Source: CAD feature listing. Evaluate the final solid. Frame: model axes, mm. A direction names the side the tool comes from. Coordinates: 2 decimals unless noted, no trailing zeros. Order: outer loops, then holes, each group sorted by start corner. A loop starts at its lowest first (then second) coordinate and runs counter-clockwise, first axis right, second up.
```python
from build123d import *

# Parameters (mm, degrees)
F0_R     = 25.4
F1_DEPTH = 635
F2_W     = 63.5
F2_H     = 50.8
F3_DEPTH = 25.4
F4_R     = 5.08


with BuildPart() as f1:
    # F0 (on Top) → F1 (new body)
    with BuildSketch(Plane.XY):
        Circle(F0_R)
    extrude(amount=F1_DEPTH)

    # F2 (on Front) → F3 (cut)
    with BuildSketch(Plane.XZ):
        with Locations((0.1835199598, 25.4)):
            Rectangle(F2_W, F2_H)
    extrude(amount=-F3_DEPTH, mode=Mode.SUBTRACT)

    # F4
    f4_edges = [f1.edges().sort_by_distance(p)[0] for p in [
        (-25.4, 0, 635),
    ]]
    fillet(f4_edges, radius=F4_R)


solid = f1.part
```
1. Pin query (flat end, axial travel): P1, Ø12, axis at y = -7.5, z = 66.5, coming from the +X side; P2, Ø4, axis at x = -20, z = 79, coming from the -Y side; P3, Ø2, axis at y = -3.5, z = 315.5, coming from the +X side. Return the tip coordinate at first contact, or that it passes through.
Findings:
P1: stops at x = 25.36
P2: stops at y = -17.92
P3: stops at x = 25.28
2. Ray query, line 1 (X direction, y = -2.5, z = 368.5); line 2 (Z direction, x = 5.5, y = -20.5); line 3 (Z direction, x = -12.5, y = 16). Return the intervals inside material, ascending.
Findings:
line 1: x = -25.28 to 25.28
line 2: z = 0 to 634.92
line 3: z = 50.8 to 635
3. Section query A-A on x = 0. Return loops of the section in (y, z), plus the area to 3 significant figures.
Findings:
outline: (-25.4, 0) - (0, 0) - (0, 50.8) - (25.4, 50.8) - (25.4, 629.92) arc R5.08 ccw to (20.32, 635) - (-20.32, 635) arc R5.08 ccw to (-25.4, 629.92) - close
area: 31,000 mm2
4. Section query B-B on z = 297. Return loops of the section in (x, y).
Findings:
outline: circle Ø50.8 at (0, 0)
5. Access query for faces 1 (the face through (0, 0, 635)), 2 (the face through (0, 0, 26)). Directions: +Z, -Z, +X, -X, +Y, -Y. A direction counts if a zero-diameter tool reaches every point of the face in a straight line with its end or side. Return the directions, or none.
Findings:
face 1: +Z, +X, -X, +Y, -Y
face 2: -Z, +X, -X, +Y
